from build123d import *

# Parameters (mm, degrees)
BOSS_EXTRUDE1_DEPTH                            = 50.8
F_8_32_TAPPED_HOLE1_D                          = 3.4544
CBORE_FOR_8_SOCKET_HEAD_CAP_SCREW1_D           = 4.4958
CBORE_FOR_8_SOCKET_HEAD_CAP_SCREW1_CBORE_D     = 7.9375
CBORE_FOR_8_SOCKET_HEAD_CAP_SCREW1_CBORE_DEPTH = 4.1656


with BuildPart() as part:
    # Sketch1 → Boss-Extrude1 (new body)
    with BuildSketch(Plane.XY):
        Polygon((25.4, 6.35), (25.4, 0), (101.6, 0), (101.6, 6.35), (76.2, 6.35), (76.2, 12.7), (0, 12.7), (0, 6.35), align=None)
    extrude(amount=BOSS_EXTRUDE1_DEPTH)

    # #8-32 Tapped Hole1 (through all)
    with Locations(Plane(origin=(0, 12.7, 0), x_dir=(1, 0, 0), z_dir=(0, 1, 0))):
        with Locations((6.35, -36.398522628), (19.05, -14.401477372)):
            Hole(F_8_32_TAPPED_HOLE1_D / 2)

    # CBORE for #8 Socket Head Cap Screw1 (through all)
    with Locations(Plane(origin=(0, 0, 0), x_dir=(-1, 0, 0), z_dir=(0, -1, 0))):
        with Locations((-95.25, -36.398522628), (-82.55, -14.401477372)):
            CounterBoreHole(CBORE_FOR_8_SOCKET_HEAD_CAP_SCREW1_D / 2, CBORE_FOR_8_SOCKET_HEAD_CAP_SCREW1_CBORE_D / 2, CBORE_FOR_8_SOCKET_HEAD_CAP_SCREW1_CBORE_DEPTH)


solid = part.part
CAD build for the part. Positions are in the model's coordinates, mm. A direction names the side the tool comes from. Give positions to 0.01 mm unless a question says otherwise; leave off trailing zeros. Write each loop counter-clockwise with the first axis right and the second up, starting at its lowest first coordinate (ties: lowest second). Pieces come first, ordered by that corner, then holes. Notation, with made-up numbers: (33, 48.5) -> (65, 48.5) arc R26 cw to (65, 85.5) -> close; hole circle Ø8 at (21, -12). An arc over 180 degrees is marked (long way). Return JSON: item names as keys, results as strings.
Item 1: Drop flat-ended pins along their axis: pin 1 (2.5 mm diameter, centred on x = 95.25, z = 36.4, fed in from +Y); pin 2 (5 mm diameter, centred on x = 74.5, z = 20, fed in from -Y); pin 3 (1 mm diameter, centred on y = 5.5, z = 6, fed in from -X); pin 4 (6.5 mm diameter, centred on x = 82.55, z = 14.4, fed in from -Y). Give the stop position or say it passes through.
Answer below:
{"pin 1": "passes through", "pin 2": "stops at y = 0", "pin 3": "stops at x = 25.4", "pin 4": "stops at y = 4.17"}
Item 2: Two-plate mould, pull along X, no slides. Class faces 5 (the flat face through (93.5, 4.166, 38.1)), 6 (the flat face through (89, 6.35, 25)), 7 (the flat face through (101.6, 3, 25)): +X half, -X half, draft (parallel to the pull), parting line (faces both ways), or undercut.
Answer below:
{"face 5": "undercut", "face 6": "draft", "face 7": "+X half"}
Item 3: Drill centre lines: probe 1 along Z at (x, y) = (6.35, 8.5); probe 2 along Z at (x, y) = (19.05, 9.75); probe 3 along X at (y, z) = (9, 44.5). Where is each one in solid material? Low to high.
Answer below:
{"probe 1": "z = 0 to 34.67, 38.13 to 50.8", "probe 2": "z = 0 to 12.67, 16.13 to 50.8", "probe 3": "x = 0 to 76.2"}
Item 4: Tool access for faces 1 (the cylindrical face through (91.465, 2.054, 35.206)), 2 (the flat face through (76.2, 9, 25)), 3 (the flat face through (25.4, 3, 25)), 4 (the flat face through (50, 6, 0)): list every direction of +Z, -Z, +X, -X, +Y, -Y with a clear straight run to the whole face (end or side of a thin tool).
Answer below:
{"face 1": "-Y", "face 2": "+Z, -Z, +X, +Y", "face 3": "+Z, -Z, -X, -Y", "face 4": "-Z, +X, -X, +Y, -Y"}
Item 5: Band-saw the part on A-A (x = 6.35). List the corners of the cut face in (y, z), then the cut area to 3 significant figures.
Answer below:
{"outline": "(6.35, 0) -> (12.7, 0) -> (12.7, 34.67) -> (6.35, 34.67) -> close; (6.35, 38.13) -> (12.7, 38.13) -> (12.7, 50.8) -> (6.35, 50.8) -> close", "area": "301 mm2"}
Item 6: Band-saw the part on B-B (z = 25). List the corners of the cut face in (x, y).
Answer below:
{"outline": "(0, 6.35) -> (25.4, 6.35) -> (25.4, 0) -> (101.6, 0) -> (101.6, 6.35) -> (76.2, 6.35) -> (76.2, 12.7) -> (0, 12.7) -> close"}
Item 7: Band-saw the part on D-D (y = 8.75). List the corners of the cut face in (x, z).
Answer below:
{"outline": "(0, 0) -> (76.2, 0) -> (76.2, 50.8) -> (0, 50.8) -> close; hole circle Ø3.45 at (6.35, 36.4); hole circle Ø3.45 at (19.05, 14.4)"}
Item 8: Band-saw the part on C-C (x = 95.25). List the corners of the cut face in (y, z), then the cut area to 3 significant figures.
Answer below:
{"outline": "(0, 0) -> (6.35, 0) -> (6.35, 34.15) -> (4.17, 34.15) -> (4.17, 32.43) -> (0, 32.43) -> close; (0, 40.37) -> (4.17, 40.37) -> (4.17, 38.65) -> (6.35, 38.65) -> (6.35, 50.8) -> (0, 50.8) -> close", "area": "280 mm2"}
